Design review of the part built by this model. Coordinates are the model's own, in mm. Face numbers are marked on the shaded views. A direction names the side the tool comes from. Give positions to 0.01 mm unless a question says otherwise; leave off trailing zeros. Write each loop counter-clockwise with the first axis right and the second up, starting at its lowest first coordinate (ties: lowest second). Pieces come first, ordered by that corner, then holes. Notation, with made-up numbers: (63.25, 31) - (94.25, 31) arc R30 ccw to (94.25, 56) - close; hole circle Ø11 at (42, 17.5). An arc over 180 degrees is marked (long way). Use a Markdown table: item, result. Add a question column.
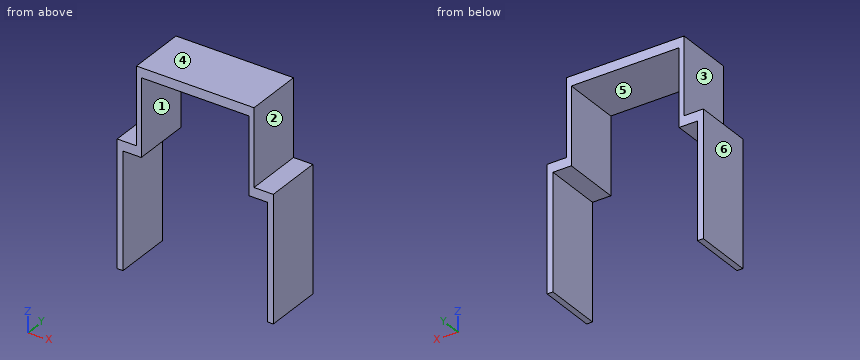
```python
from build123d import *

# Parameters (mm, degrees)
ESQUISSE1_W             = 61
ESQUISSE1_H             = 30
BOSS_EXTRU_1_DEPTH      = 45
ESQUISSE2_W             = 56
ESQUISSE2_H             = 30
ENL_V_MAT_EXTRU_1_DEPTH = 40
ESQUISSE3_W             = 5
ESQUISSE3_H             = 30
BOSS_EXTRU_2_DEPTH      = 10
ESQUISSE4_W             = 5
ESQUISSE4_H             = 30
BOSS_EXTRU_3_DEPTH      = 10
ESQUISSE5_W             = 3
ESQUISSE5_H             = 30
BOSS_EXTRU_4_DEPTH      = 60
ESQUISSE6_W             = 3
ESQUISSE6_H             = 30
BOSS_EXTRU_5_DEPTH      = 60


with BuildPart() as part:
    # Esquisse1 → Boss.-Extru.1 (new body)
    with BuildSketch(Plane.XY):
        with Locations((-2.408366894, 0.644052045)):
            Rectangle(ESQUISSE1_W, ESQUISSE1_H)
    extrude(amount=BOSS_EXTRU_1_DEPTH)

    # Esquisse2 → Enlèv. mat.-Extru.1 (cut)
    with BuildSketch(Plane(origin=(0, 0, 0), x_dir=(-1, 0, 0), z_dir=(0, 0, -1))):
        with Locations((2.408366894, 0.644052045)):
            Rectangle(ESQUISSE2_W, ESQUISSE2_H)
    extrude(amount=-ENL_V_MAT_EXTRU_1_DEPTH, mode=Mode.SUBTRACT)

    # Esquisse3 → Boss.-Extru.2 (add)
    with BuildSketch(Plane(origin=(28.091633106, 0, 0), x_dir=(0, 0, -1), z_dir=(1, 0, 0))):
        with Locations((-2.5, 0.644052045)):
            Rectangle(ESQUISSE3_W, ESQUISSE3_H)
    extrude(amount=BOSS_EXTRU_2_DEPTH)

    # Esquisse4 → Boss.-Extru.3 (add)
    with BuildSketch(Plane.ZY.offset(32.908366894)):
        with Locations((2.5, 0.644052045)):
            Rectangle(ESQUISSE4_W, ESQUISSE4_H)
    extrude(amount=BOSS_EXTRU_3_DEPTH)

    # Esquisse5 → Boss.-Extru.4 (add)
    with BuildSketch(Plane(origin=(0, 0, 0), x_dir=(-1, 0, 0), z_dir=(0, 0, -1))):
        with Locations((-36.591633106, 0.644052045)):
            Rectangle(ESQUISSE5_W, ESQUISSE5_H)
    extrude(amount=BOSS_EXTRU_4_DEPTH)

    # Esquisse6 → Boss.-Extru.5 (add)
    with BuildSketch(Plane(origin=(0, 0, 0), x_dir=(-1, 0, 0), z_dir=(0, 0, -1))):
        with Locations((41.408366894, 0.644052045)):
            Rectangle(ESQUISSE6_W, ESQUISSE6_H)
    extrude(amount=BOSS_EXTRU_5_DEPTH)


solid = part.part
```
(1) Insertion check: pin 1 (11 mm diameter, centred on x = 31.5, y = 1.5, fed in from +Z); pin 2 (15 mm diameter, centred on y = 5.5, z = 20, fed in from +X); pin 3 (5 mm diameter, centred on x = 31, y = 5, fed in from -Z); pin 4 (15 mm diameter, centred on y = -0.5, z = 18, fed in from -X). Each pin has a flat end and moves straight along its axis. Give the tip position at first contact, or say it passes through.
(2) Add section A-A (z = 37). State the section outline as (x, y) points, and give its area (3 significant figures).
(3) Add section B-B (z = -5). State the section outline as (x, y) points, and give its area (3 significant figures).
(4) Tool access review of the marked faces 1, 2 and 3: name each direction out of +Z, -Z, +X, -X, +Y, -Y from which nothing blocks a thin tool from reaching the whole face with its end or side.
(5) Mouldability with a two-part tool opening along X and no side actions: class the marked faces 4, 5 and 6 as +X half, -X half, draft (parallel to the pull), parting line (faces both ways), or undercut.
(6) For line 1 along X through (y, z) = (-2, -42); line 2 along X through (y, z) = (6, 21); line 3 along Z through (x, y) = (-14.5, 6), list the stretches that pass through material, from the lowest coordinate up.
(7) Add section D-D (x = -16). State the section outline as (y, z) points, and give its area (3 significant figures).
(8) Add section C-C (y = 2.75). State the section outline as (x, z) points.
Answers follow:
| question | item | result |
|---|---|---|
| 1 | pin 1 | z = 45 |
| 1 | pin 2 | x = 28.09 |
| 1 | pin 3 | z = 0 |
| 1 | pin 4 | x = -32.91 |
| 2 | outline | (-32.91, -14.36) - (-30.41, -14.36) - (-30.41, 15.64) - (-32.91, 15.64) - close; (25.59, -14.36) - (28.09, -14.36) - (28.09, 15.64) - (25.59, 15.64) - close |
| 2 | area | 150 mm^2 |
| 3 | outline | (-42.91, -14.36) - (-39.91, -14.36) - (-39.91, 15.64) - (-42.91, 15.64) - close; (35.09, -14.36) - (38.09, -14.36) - (38.09, 15.64) - (35.09, 15.64) - close |
| 3 | area | 180 mm^2 |
| 4 | face 1 | -Z, +Y, -Y |
| 4 | face 2 | +Z, +X, +Y, -Y |
| 4 | face 3 | +Z, -X, +Y, -Y |
| 5 | face 4 | draft |
| 5 | face 5 | undercut |
| 5 | face 6 | -X half |
| 6 | line 1 | -42.91 to -39.91, 35.09 to 38.09 |
| 6 | line 2 | -32.91 to -30.41, 25.59 to 28.09 |
| 6 | line 3 | 40 to 45 |
| 7 | outline | (-14.36, 40) - (15.64, 40) - (15.64, 45) - (-14.36, 45) - close |
| 7 | area | 150 mm^2 |
| 8 | outline | (-42.91, -60) - (-39.91, -60) - (-39.91, 0) - (-30.41, 0) - (-30.41, 40) - (25.59, 40) - (25.59, 0) - (35.09, 0) - (35.09, -60) - (38.09, -60) - (38.09, 5) - (28.09, 5) - (28.09, 45) - (-32.91, 45) - (-32.91, 5) - (-42.91, 5) - close |
